The model under review builds one solid part; all positions refer to its coordinate system, in mm. A direction names the side the tool comes from. Round coordinates to 2 decimals unless told otherwise and drop trailing zeros. Order: outer loops, then holes, each group sorted by start corner. A loop starts at its lowest first (then second) coordinate and runs counter-clockwise, first axis right, second up. Notation, with made-up numbers: M 25,63 L 35,63 A34 cw 35,102 Z; hole C -36.75,37.25 d5. An arc over 180 degrees is marked long. Answer as a JSON object with one key per item and string values. Group by question number.
1) The part is to be moulded in two halves that separate along Y. For faces 1 (the flat face through (-98, 97, 3)), 2 (the flat face through (-79, 110, 3)), 3 (the flat face through (-158.3, 1.7, 3)), say which applies: +Y half, -Y half, draft (parallel to the pull), parting line (faces both ways), or undercut.
2) Insertion check: pin 1 Ø4 at (x, y) = (-13, 3) entering from -Z; pin 2 Ø2 at (x, z) = (-102, 3.5) entering from -Y; pin 3 Ø3 at (x, z) = (-136, 2.5) entering from +Y. Each pin has a flat end and moves straight along its axis. Give the tip position at first contact, or say it passes through.
3) Consider section C-C, the plane z = 4.25. Count the separate pieces of the cut face and the enclosed holes in it, then the cut area to 3 significant figures.
4) Consider section D-D, the plane x = -186.5. Write out the cut boundary in (y, z).
5) To check wall thickness, follow line 1 (X direction, y = 69.5, z = 0.95); line 2 (X direction, y = 66.5, z = 5.1); line 3 (X direction, y = 98.5, z = 0.55). State the ranges of each line that lie inside material, in increasing order.
6) Consider section B-B, the plane y = 61. Write out the cut boundary in (x, z).
7) Consider section A-A, the plane y = 97.5. Write out the cut boundary in (x, z), then the cut area to 3 significant figures.
8) For faces 4 (the flat face through (-164, 3, 3)), 5 (the flat face through (-135, 104, 3)), 6 (the cylindrical face through (-15.857, 3.9, 1.479)), 7 (the flat face through (-270, 107, 3)), list the 3-axis set-ups (+Z, -Z, +X, -X, +Y, -Y) from which the entire face can be reached by the end or side of a thin tool; tool diameter is ignored.
```python
from build123d import *

# Parameters (mm, degrees)
ESQUISSE2_W             = 330
ESQUISSE2_H             = 110
BOSS_EXTRU_1_DEPTH      = 6
ESQUISSE3_W             = 6
ESQUISSE3_H             = 37
ESQUISSE3_W_2           = 60
ESQUISSE3_H_2           = 6
ESQUISSE3_H_3           = 30
ESQUISSE3_H_4           = 39
ESQUISSE3_W_3           = 3
ENL_V_MAT_EXTRU_1_DEPTH = 348.902285132
ESQUISSE4_W             = 56.799161249
ESQUISSE4_H             = 104
ENL_V_MAT_EXTRU_2_DEPTH = 348.902285132
ESQUISSE5_R             = 1.5
ENL_V_MAT_EXTRU_3_DEPTH = 301.892007205
ESQUISSE6_R             = 2.995
ENL_V_MAT_EXTRU_5_DEPTH = 3


with BuildPart() as part:
    # Esquisse2 → Boss.-Extru.1 (new body)
    with BuildSketch(Plane.XY):
        with Locations((-165, 55)):
            Rectangle(ESQUISSE2_W, ESQUISSE2_H)
    extrude(amount=BOSS_EXTRU_1_DEPTH)

    # Esquisse3 → Enlèv. mat.-Extru.1 (cut, through all)
    with BuildSketch(Plane.XY.offset(6)):
        Polygon((-60, 110), (0, 110), (0, 57), (-6, 57), (-6, 104), (-20, 104), (-20, 84), (-60, 84), align=None)
        with Locations((-3, 18.5)):
            Rectangle(ESQUISSE3_W, ESQUISSE3_H)
        Polygon((-330, 110), (-270, 110), (-270, 104), (-324, 104), (-324, 59), (-330, 59), align=None)
        with Locations((-86, 3)):
            Rectangle(ESQUISSE3_W_2, ESQUISSE3_H_2)
        with Locations((-194, 3)):
            Rectangle(ESQUISSE3_W_2, ESQUISSE3_H_2)
        with Locations((-277, 53.5)):
            Rectangle(ESQUISSE3_W, ESQUISSE3_H_3)
        with Locations((-327, 19.5)):
            Rectangle(ESQUISSE3_W, ESQUISSE3_H_4)
        Polygon((-98, 110), (-98, 84), (-128, 84), (-128, 104), (-142, 104), (-142, 74), (-162, 74), (-162, 104), (-232, 104), (-232, 110), align=None)
        with Locations((-133.5, 59.5)):
            Rectangle(ESQUISSE3_W_3, ESQUISSE3_H_3)
    extrude(amount=-ENL_V_MAT_EXTRU_1_DEPTH, mode=Mode.SUBTRACT)

    # Esquisse4 → Enlèv. mat.-Extru.2 (cut, through all)
    with BuildSketch(Plane.XY.offset(6)):
        with Locations((-308.399580625, 52)):
            Rectangle(ESQUISSE4_W, ESQUISSE4_H)
    extrude(amount=-ENL_V_MAT_EXTRU_2_DEPTH, mode=Mode.SUBTRACT)

    # Esquisse5 → Enlèv. mat.-Extru.3 (cut, through all)
    with BuildSketch(Plane(origin=(0, 0, 0), x_dir=(-1, 0, 0), z_dir=(0, 0, -1))):
        with Locations((13, 3)):
            Circle(ESQUISSE5_R)
        with Locations((49, 3)):
            Circle(ESQUISSE5_R)
        with Locations((123, 3)):
            Circle(ESQUISSE5_R)
        with Locations((157, 3)):
            Circle(ESQUISSE5_R)
        with Locations((231, 3)):
            Circle(ESQUISSE5_R)
        with Locations((273, 3)):
            Circle(ESQUISSE5_R)
    extrude(amount=-ENL_V_MAT_EXTRU_3_DEPTH, mode=Mode.SUBTRACT)

    # Esquisse6 → Enlèv. mat.-Extru.5 (cut)
    with BuildSketch(Plane(origin=(0, 0, 0), x_dir=(-1, 0, 0), z_dir=(0, 0, -1))):
        with Locations((13, 3)):
            Circle(ESQUISSE6_R)
        with Locations((49, 3)):
            Circle(ESQUISSE6_R)
        with Locations((123, 3)):
            Circle(ESQUISSE6_R)
        with Locations((157, 3)):
            Circle(ESQUISSE6_R)
        with Locations((273, 3)):
            Circle(ESQUISSE6_R)
        with Locations((231, 3)):
            Circle(ESQUISSE6_R)
    extrude(amount=-ENL_V_MAT_EXTRU_5_DEPTH, mode=Mode.SUBTRACT)


solid = part.part
```
Results list:
{
 "1": {"face 1": "draft", "face 2": "+Y half", "face 3": "undercut"},
 "2": {"pin 1": "z = 3", "pin 2": "y = 6", "pin 3": "y = 104"},
 "3": {"separate pieces": "1", "enclosed holes": "7", "area": "26,000 mm^2"},
 "4": {"outline": "M 6,0 L 104,0 L 104,6 L 6,6 Z"},
 "5": {"line 1": "-280 to -135, -132 to -6", "line 2": "-274 to -135, -132 to -6", "line 3": "-280 to -162, -142 to -128, -98 to -60, -20 to -6"},
 "6": {"outline": "M -274,0 L -135,0 L -135,6 L -274,6 Z; M -132,0 L -6,0 L -6,6 L -132,6 Z"},
 "7": {"outline": "M -280,0 L -162,0 L -162,6 L -280,6 Z; M -142,0 L -128,0 L -128,6 L -142,6 Z; M -98,0 L -60,0 L -60,6 L -98,6 Z; M -20,0 L -6,0 L -6,6 L -20,6 Z", "area": "1,100 mm^2"},
 "8": {"face 4": "+Z, -Z, -Y", "face 5": "+Z, -Z, +Y", "face 6": "-Z", "face 7": "+Z, -Z, -X, +Y"}
}
